Here's how the part is built. I have some questions about the finished solid (model axes, mm). Give positions to 0.01 mm unless a question says otherwise; leave off trailing zeros. Write each loop counter-clockwise with the first axis right and the second up, starting at its lowest first coordinate (ties: lowest second). Pieces come first, ordered by that corner, then holes. Notation, with made-up numbers: (-9.75, -18) - (-0.75, -18) arc R5 ccw to (-0.75, -14) - close; hole circle Ø8 at (55, -19.75). An arc over 180 degrees is marked (long way). Use a Markdown table: item, result.
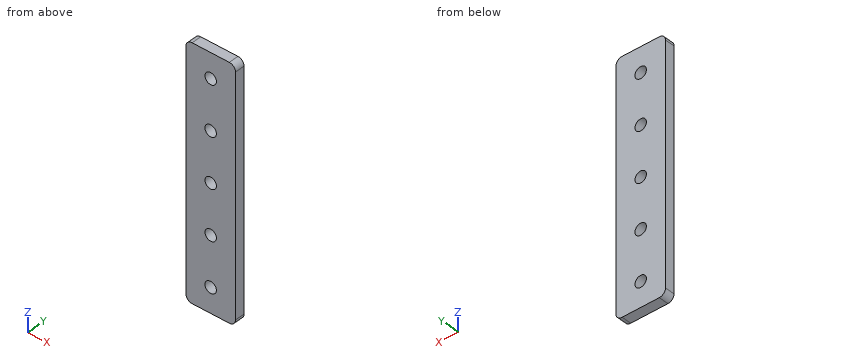
```python
from build123d import *

# Parameters (mm, degrees)
SKETCH1_R               = 1.85
BOSS_EXTRUDE1_DEPTH     = 3.2
CUT_EXTRUDE1_DEPTH      = 4.2
CUT_EXTRUDE1_DEPTH_BACK = 1
FILLET1_R               = 2


with BuildPart() as part:
    # Sketch1 → Boss-Extrude1 (new body)
    with BuildSketch(Plane(origin=(0, 3.2, 0), x_dir=(1, 0, 0), z_dir=(0, 1, 0))):
        with BuildLine():
            Line((8, 2), (8, 286))
            ThreePointArc((8, 286), (7.414213562, 287.414213562), (6, 288))
            Line((6, 288), (-6, 288))
            ThreePointArc((-6, 288), (-7.414213562, 287.414213562), (-8, 286))
            Line((-8, 286), (-8, 2))
            ThreePointArc((-8, 2), (-7.414213562, 0.585786438), (-6, 0))
            Line((-6, 0), (6, 0))
            ThreePointArc((6, 0), (7.414213562, 0.585786438), (8, 2))
        make_face()
        with Locations((0, 280)):
            Circle(SKETCH1_R, mode=Mode.SUBTRACT)
        with Locations((0, 264)):
            Circle(SKETCH1_R, mode=Mode.SUBTRACT)
        with Locations((0, 248)):
            Circle(SKETCH1_R, mode=Mode.SUBTRACT)
        with Locations((0, 232)):
            Circle(SKETCH1_R, mode=Mode.SUBTRACT)
        with Locations((0, 216)):
            Circle(SKETCH1_R, mode=Mode.SUBTRACT)
        with Locations((0, 200)):
            Circle(SKETCH1_R, mode=Mode.SUBTRACT)
        with Locations((0, 184)):
            Circle(SKETCH1_R, mode=Mode.SUBTRACT)
        with Locations((0, 168)):
            Circle(SKETCH1_R, mode=Mode.SUBTRACT)
        with Locations((0, 152)):
            Circle(SKETCH1_R, mode=Mode.SUBTRACT)
        with Locations((0, 136)):
            Circle(SKETCH1_R, mode=Mode.SUBTRACT)
        with Locations((0, 120)):
            Circle(SKETCH1_R, mode=Mode.SUBTRACT)
        with Locations((0, 104)):
            Circle(SKETCH1_R, mode=Mode.SUBTRACT)
        with Locations((0, 88)):
            Circle(SKETCH1_R, mode=Mode.SUBTRACT)
        with Locations((0, 72)):
            Circle(SKETCH1_R, mode=Mode.SUBTRACT)
        with Locations((0, 56)):
            Circle(SKETCH1_R, mode=Mode.SUBTRACT)
        with Locations((0, 40)):
            Circle(SKETCH1_R, mode=Mode.SUBTRACT)
        with Locations((0, 24)):
            Circle(SKETCH1_R, mode=Mode.SUBTRACT)
        with Locations((0, 8)):
            Circle(SKETCH1_R, mode=Mode.SUBTRACT)
    extrude(amount=-BOSS_EXTRUDE1_DEPTH)

    # Sketch2 → Cut-Extrude1 (cut, two sides)
    with BuildSketch(Plane(origin=(0, 0, 0), x_dir=(1, 0, 0), z_dir=(0, 1, 0))) as cut_extrude1_sk:
        Polygon((-474.979607439, 80), (-38.646772996, 80), (26.442528892, 80), (462.775363335, 80), (462.775363335, 952.665668885), (-474.979607439, 952.665668885), align=None)
    extrude(amount=CUT_EXTRUDE1_DEPTH, mode=Mode.SUBTRACT)
    extrude(cut_extrude1_sk.sketch, amount=-CUT_EXTRUDE1_DEPTH_BACK, mode=Mode.SUBTRACT)

    # Fillet1
    fillet1_edges = [part.edges().sort_by_distance(p)[0] for p in [
        (8, 1.6, -80),
        (-8, 1.6, -80),
    ]]
    fillet(fillet1_edges, radius=FILLET1_R)


solid = part.part
```
Item 1: I need wall thicknesses on line 1 along Z through (x, y) = (0, 2.5); line 2 along X through (y, z) = (0.8, -8); line 3 along Z through (x, y) = (-6.25, 1.4). Which ranges of each line are inside material? Lowest first, please. Write a range as [from, to].
Values:
| item | result |
|---|---|
| line 1 | z = [-80, -73.85], [-70.15, -57.85], [-54.15, -41.85], [-38.15, -25.85], [-22.15, -9.85], [-6.15, 0] |
| line 2 | x = [-8, -1.85], [1.85, 8] |
| line 3 | z = [-79.98, -0.02] |
Item 2: If we section it at A-A, the plane z = -40: Write out the boundary of the cut face in (x, y).
Values:
| item | result |
|---|---|
| outline | (-8, 0) - (-1.85, 0) - (-1.85, 3.2) - (-8, 3.2) - close; (1.85, 0) - (8, 0) - (8, 3.2) - (1.85, 3.2) - close |
Item 3: If we section it at C-C, the plane x = 0: Write out the boundary of the cut face in (y, z).
Values:
| item | result |
|---|---|
| outline | (0, -80) - (3.2, -80) - (3.2, -73.85) - (0, -73.85) - close; (0, -70.15) - (3.2, -70.15) - (3.2, -57.85) - (0, -57.85) - close; (0, -54.15) - (3.2, -54.15) - (3.2, -41.85) - (0, -41.85) - close; (0, -38.15) - (3.2, -38.15) - (3.2, -25.85) - (0, -25.85) - close; (0, -22.15) - (3.2, -22.15) - (3.2, -9.85) - (0, -9.85) - close; (0, -6.15) - (3.2, -6.15) - (3.2, 0) - (0, 0) - close |
Item 4: Will this pin go through, and if not, where does the flat tip stop? pin 1 Ø3.5 at (x, z) = (0, -72) entering from +Y.
Values:
| item | result |
|---|---|
| pin 1 | passes through |
Item 5: If we section it at D-D, the plane z = -23: Write out the boundary of the cut face in (x, y), plus the area to 3 significant figures.
Values:
| item | result |
|---|---|
| outline | (-8, 0) - (-1.56, 0) - (-1.56, 3.2) - (-8, 3.2) - close; (1.56, 0) - (8, 0) - (8, 3.2) - (1.56, 3.2) - close |
| area | 41.2 mm2 |
Item 6: If we section it at B-B, the plane y = 2.1: Write out the boundary of the cut face in (x, z).
Values:
| item | result |
|---|---|
| outline | (-8, -78) arc R2 ccw to (-6, -80) - (6, -80) arc R2 ccw to (8, -78) - (8, -2) arc R2 ccw to (6, 0) - (-6, 0) arc R2 ccw to (-8, -2) - close; hole circle Ø3.7 at (0, -72); hole circle Ø3.7 at (0, -56); hole circle Ø3.7 at (0, -40); hole circle Ø3.7 at (0, -24); hole circle Ø3.7 at (0, -8) |
